The drawing under review shows one solid part. Ordinate dimensions are in mm from its lowest x, y, z. Round coordinates to 2 decimals unless told otherwise and drop trailing zeros. Loops run counter-clockwise (first coordinate to the right, second up) from the corner with the lowest first, then second, coordinate; pieces in that order, holes last. Notation, with made-up numbers: (25.5, -20) -> (69.5, -20) arc R15 ccw to (69.5, 3) -> close; hole circle Ø5 at (47, -32.5). An arc over 180 degrees is marked (long way). Answer as CSV lines item,"result". Start each with the question number.
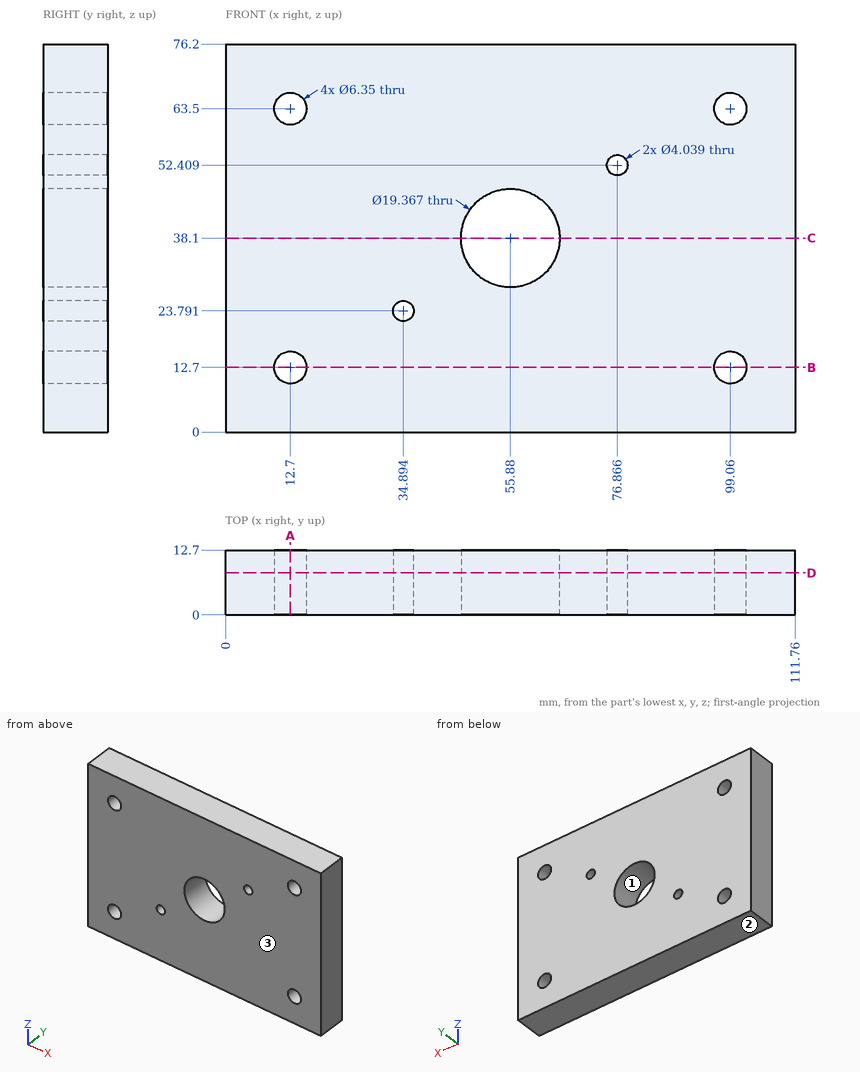
Q1. Add section A-A, the plane x = 12.7. Give the boundary of the cut face in (y, z) (1 decimal).
Q2. For pin 1 Ø2.5 at (x, z) = (76.87, 52.41) entering from +Y, flat-tipped, find the tip position at first contact; note if it passes through.
Q3. Mouldability with a two-part tool opening along Z and no side actions: class the marked faces 1, 2 and 3 as pulls with the +Z half, pulls with the -Z half, needs draft (parallel to the pull), parting line crosses it, or undercut.
Q4. To check wall thickness, follow probe 1 along Z at (x, y) = (12.7, 7.25) (1 decimal); probe 2 along X at (y, z) = (3, 63.5) (1 decimal); probe 3 along Z at (x, y) = (55.88, 6.25). State the ranges of each line that lie inside material, in increasing order. Write a range as from..to.
Q5. Add section B-B, the plane z = 12.7. Give the boundary of the cut face in (x, y) (1 decimal).
Q6. Add section C-C, the plane z = 38.1. Give the boundary of the cut face in (x, y).
Q7. Add section D-D, the plane y = 8.25. State how many separate pieces and enclosed holes the cut face has, and give its area (3 significant figures).
Worked answers:
1,outline,"(0, 0) -> (12.7, 0) -> (12.7, 9.5) -> (0, 9.5) -> close; (0, 15.9) -> (12.7, 15.9) -> (12.7, 60.3) -> (0, 60.3) -> close; (0, 66.7) -> (12.7, 66.7) -> (12.7, 76.2) -> (0, 76.2) -> close"
2,pin 1,"passes through"
3,face 1,"undercut"
3,face 2,"pulls with the -Z half"
3,face 3,"needs draft"
4,probe 1,"z = 0..9.5, 15.9..60.3, 66.7..76.2"
4,probe 2,"x = 0..9.5, 15.9..95.9, 102.2..111.8"
4,probe 3,"z = 0..28.42, 47.78..76.2"
5,outline,"(0, 0) -> (9.5, 0) -> (9.5, 12.7) -> (0, 12.7) -> close; (15.9, 0) -> (95.9, 0) -> (95.9, 12.7) -> (15.9, 12.7) -> close; (102.2, 0) -> (111.8, 0) -> (111.8, 12.7) -> (102.2, 12.7) -> close"
6,outline,"(0, 0) -> (46.2, 0) -> (46.2, 12.7) -> (0, 12.7) -> close; (65.56, 0) -> (111.76, 0) -> (111.76, 12.7) -> (65.56, 12.7) -> close"
7,separate pieces,"1"
7,enclosed holes,"7"
7,area,"8,070 mm^2"
